```python
from build123d import *

# Parameters (mm, degrees)
F0_R     = 22.5
F0_R_2   = 10
F1_DEPTH = 10
F4_DEPTH = 10
F5_R     = 25
F6_R     = 5
F7_R     = 20


with BuildPart() as f1:
    # F0 (on Top) → F1 (new body)
    with BuildSketch(Plane.XY):
        Circle(F0_R)
        Circle(F0_R_2, mode=Mode.SUBTRACT)
    extrude(amount=-F1_DEPTH)

    # F3 (on offset) → F4 (join)
    with BuildSketch(Plane.XZ.offset(-22.5)):
        with BuildLine():
            Line((0, -20), (0, 0))
            Line((0, 0), (-58.776934, 0))
            Line((-58.776934, 0), (-93.19152, -49.149123))
            ThreePointArc((-93.19152, -49.149123), (-94.848078, -56.621369), (-90.735764, -63.076407))
            ThreePointArc((-90.735764, -63.076407), (-83.263518, -64.732965), (-76.80848, -60.620651))
            Line((-76.80848, -60.620651), (-48.365593, -20))
            Line((-48.365593, -20), (0, -20))
        make_face()
        with BuildLine():
            Line((-57.059605, -21.955655), (-81.723392, -57.179193))
            ThreePointArc((-81.723392, -57.179193), (-87.294306, -58.161495), (-88.276608, -52.590581))
            Line((-88.276608, -52.590581), (-63.612821, -17.367043))
            ThreePointArc((-63.612821, -17.367043), (-58.041907, -16.384741), (-57.059605, -21.955655))
        make_face(mode=Mode.SUBTRACT)
    extrude(amount=F4_DEPTH)

    # F5
    f5_edges = [f1.edges().sort_by_distance(p)[0] for p in [
        (-58.776934, 17.5, 0),
    ]]
    fillet(f5_edges, radius=F5_R)

    # F6
    f6_edges = [f1.edges().sort_by_distance(p)[0] for p in [
        (-48.365593, 17.5, -20),
    ]]
    fillet(f6_edges, radius=F6_R)

    # F7
    f7_edges = [f1.edges().sort_by_distance(p)[0] for p in [
        (-18.708287, 12.5, -5),
    ]]
    fillet(f7_edges, radius=F7_R)


solid = f1.part
```
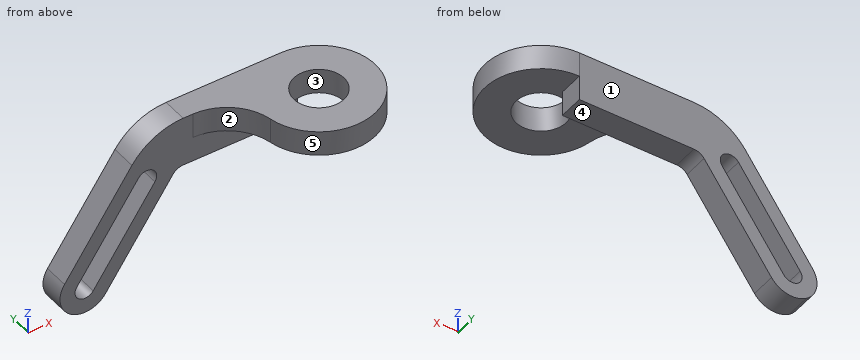
Here's how the part is built. I have some questions about the finished solid (model axes, mm). Face numbers are marked on the shaded views. A direction names the side the tool comes from. Coordinates: 2 decimals unless noted, no trailing zeros. Order: outer loops, then holes, each group sorted by start corner. A loop starts at its lowest first (then second) coordinate and runs counter-clockwise, first axis right, second up. Notation, with made-up numbers: (4.25, 89) - (21.25, 89) arc R27 cw to (21.25, 121) - close; hole circle Ø10 at (84.25, 29). An arc over 180 degrees is marked (long way). One line per question, with ' | ' between items. Start each with the question number.
1. Please list where these lines run through material, in increasing order: line 1 along Y through (x, z) = (0, -4); line 2 along Z through (x, y) = (-3, 17.5); line 3 along Z through (x, y) = (11.5, 12.5). Write a range as [from, to].
2. I'm going to push flat-ended pins straight in: pin 1 Ø2 at (y, z) = (13.5, -10) entering from -X; pin 2 Ø19.5 at (x, z) = (-42.5, -19) entering from -Y; pin 3 Ø11 at (y, z) = (19.5, -17.5) entering from +X. Where does each tip first touch, or does it pass through?
3. If we section it at D-D (x = -38): Write out the boundary of the cut face in (y, z), and give its area (3 significant figures).
4. Which directions (+Z, -Z, +X, -X, +Y, -Y) give clear straight access to the entire face, cutting with the end or side of a thin tool? Please do the marked faces 4 and 5.
5. If we section it at C-C (z = -5.5): Write out the boundary of the cut face in (x, y).
6. If we section it at B-B (y = 0): Write out the boundary of the cut face in (x, z).
7. If we section it at A-A (x = -85): Write out the boundary of the cut face in (y, z).
8. If we mould it in two halves opening along X, with no side actions, what happens to the marked faces 1, 2 and 3? For each: released by +X, released by -X, zero draft, split by the parting line, or undercut.
Model answer:
1) line 1: y = [-22.5, -10], [10, 22.5] | line 2: z = [-20, 0] | line 3: z = [-10, 0]
2) pin 1: stops at x = -66.48 | pin 2: stops at y = 12.26 | pin 3: stops at x = 0
3) outline: (12.13, -10) - (12.5, -10) - (12.5, -20) - (22.5, -20) - (22.5, 0) - (12.13, 0) - close | area: 204 mm²
4) face 4: -Z, +X, +Y, -Y | face 5: +Z, -Z
5) outline: (-61.41, 12.5) - (-41.83, 12.5) arc R20 cw to (-22.15, -3.97) arc R22.5 ccw (long way) to (0, 22.5) - (-61.41, 22.5) - close; hole circle Ø20 at (0, 0)
6) outline: (-23.29, -10) - (-10, -10) - (-10, 0) - (-23.29, 0) - close; (10, -10) - (22.5, -10) - (22.5, 0) - (10, 0) - close
7) outline: (12.5, -64.88) - (22.5, -64.88) - (22.5, -58.88) - (12.5, -58.88) - close; (12.5, -47.91) - (22.5, -47.91) - (22.5, -37.45) - (12.5, -37.45) - close
8) face 1: zero draft | face 2: released by -X | face 3: undercut
